Here's how the part is built. I have some questions about the finished solid (model axes, mm). A direction names the side the tool comes from. Give positions to 0.01 mm unless a question says otherwise; leave off trailing zeros. Loops run counter-clockwise (first coordinate to the right, second up) from the corner with the lowest first, then second, coordinate; pieces in that order, holes last.
Q1. Suppose I cut it at D-D (z = 15.75). List the corners of the cut face in (x, y) for me.
Q2. Suppose I cut it at C-C (z = 4). List the corners of the cut face in (x, y) for me.
Q3. Suppose I cut it at B-B (x = 5.5). List the corners of the cut face in (y, z) for me.
Q4. I'm going to push flat-ended pins straight in: P1, Ø1, axis at x = 23, z = 12.5, coming from the -Y side; P2, Ø2, axis at y = 34, z = 14, coming from the -X side; P3, Ø12, axis at y = 33.5, z = 11.5, coming from the +X side; P4, Ø4, axis at x = 5.5, y = 39.1, coming from the -Z side. Where does each tip first touch, or does it pass through?
Q5. Thinking about a two-plate mould opening in Y: for faces 1 (the face through (35, 59, 12)), 2 (the face through (35, 56, 12)), 3 (the face through (70, 35, 2)), which applies, pulls with the +Y half, pulls with the -Y half, needs draft (parallel to the pull), parting line crosses it, or undercut?
Q6. For faces 4 (the face through (59, 35, 12)), 5 (the face through (31, 12, 13)), 6 (the face through (11, 35, 12)), which set-ups out of +Z, -Z, +X, -X, +Y, -Y let a thin tool reach every point of the face, with its end or its side?
Q7. I need wall thicknesses on probe 1 along Y at (x, z) = (5.5, 1); probe 2 along X at (y, z) = (22.5, 5.25); probe 3 along Y at (x, z) = (30.9, 3.4). Which ranges of each line are inside material? Lowest first, please.
Q8. Suppose I cut it at A-A (y = 39.1). List the corners of the cut face in (x, z) for me.
```python
from build123d import *

# Parameters (mm, degrees)
SKETCH1_W          = 70
SKETCH1_H          = 70
EXTRUDE1_DEPTH     = 5
SKETCH2_W          = 48
SKETCH2_H          = 48
SKETCH2_W_2        = 42
SKETCH2_H_2        = 42
EXTRUDE2_DEPTH     = 15
SKETCH5_R          = 3.25
CUT_EXTRUDE2_DEPTH = 101.124921973
SKETCH6_W          = 8
SKETCH6_H          = 8
CUT_EXTRUDE3_DEPTH = 15


with BuildPart() as part:
    # Sketch1 → Extrude1 (new body)
    with BuildSketch(Plane.XY):
        with Locations((35, 35)):
            Rectangle(SKETCH1_W, SKETCH1_H)
    extrude(amount=EXTRUDE1_DEPTH)

    # Sketch2 → Extrude2 (add)
    with BuildSketch(Plane.XY.offset(5)):
        with Locations((35, 35)):
            Rectangle(SKETCH2_W, SKETCH2_H)
        with Locations((35, 35)):
            Rectangle(SKETCH2_W_2, SKETCH2_H_2, mode=Mode.SUBTRACT)
    extrude(amount=EXTRUDE2_DEPTH)

    # Sketch5 → Cut-Extrude2 (cut, through all)
    with BuildSketch(Plane.XY.offset(5)):
        with Locations((5.5, 64.5)):
            Circle(SKETCH5_R)
        with Locations((30.9, 64.5)):
            Circle(SKETCH5_R)
        with Locations((56.3, 64.5)):
            Circle(SKETCH5_R)
        with Locations((5.5, 39.1)):
            Circle(SKETCH5_R)
        with Locations((5.5, 13.7)):
            Circle(SKETCH5_R)
    extrude(amount=-CUT_EXTRUDE2_DEPTH, mode=Mode.SUBTRACT)

    # Sketch6 → Cut-Extrude3 (cut)
    with BuildSketch(Plane.XY.offset(20)):
        with Locations((35, 14)):
            Rectangle(SKETCH6_W, SKETCH6_H)
    extrude(amount=-CUT_EXTRUDE3_DEPTH, mode=Mode.SUBTRACT)


solid = part.part
```
Solutions:
1. outline: (11, 11) - (31, 11) - (31, 14) - (14, 14) - (14, 56) - (56, 56) - (56, 14) - (39, 14) - (39, 11) - (59, 11) - (59, 59) - (11, 59) - close
2. outline: (0, 0) - (70, 0) - (70, 70) - (0, 70) - close; hole circle Ø6.5 at (5.5, 13.7); hole circle Ø6.5 at (5.5, 39.1); hole circle Ø6.5 at (5.5, 64.5); hole circle Ø6.5 at (30.9, 64.5); hole circle Ø6.5 at (56.3, 64.5)
3. outline: (0, 0) - (10.45, 0) - (10.45, 5) - (0, 5) - close; (16.95, 0) - (35.85, 0) - (35.85, 5) - (16.95, 5) - close; (42.35, 0) - (61.25, 0) - (61.25, 5) - (42.35, 5) - close; (67.75, 0) - (70, 0) - (70, 5) - (67.75, 5) - close
4. P1: stops at y = 11
4. P2: stops at x = 11
4. P3: stops at x = 59
4. P4: passes through
5. face 1: pulls with the +Y half
5. face 2: undercut
5. face 3: needs draft
6. face 4: +Z, +X, +Y, -Y
6. face 5: +Z, -Y
6. face 6: +Z, -X, +Y, -Y
7. probe 1: y = 0 to 10.45, 16.95 to 35.85, 42.35 to 61.25, 67.75 to 70
7. probe 2: x = 11 to 14, 56 to 59
7. probe 3: y = 0 to 61.25, 67.75 to 70
8. outline: (0, 0) - (2.25, 0) - (2.25, 5) - (0, 5) - close; (8.75, 0) - (70, 0) - (70, 5) - (59, 5) - (59, 20) - (56, 20) - (56, 5) - (14, 5) - (14, 20) - (11, 20) - (11, 5) - (8.75, 5) - close
